```python
from build123d import *

# Parameters (mm, degrees)
SKETCH1_W           = 31
SKETCH1_H           = 16.5
BOSS_EXTRUDE1_DEPTH = 13
SKETCH2_W           = 21
SKETCH2_H           = 1.75
CUT_EXTRUDE1_DEPTH  = 1.6


with BuildPart() as part:
    # Sketch1 → Boss-Extrude1 (new body)
    with BuildSketch(Plane(origin=(0, 0, 0), x_dir=(1, 0, 0), z_dir=(0, 1, 0))):
        Rectangle(SKETCH1_W, SKETCH1_H)
        Polygon((10.5, 5), (-10.5, 5), (-10.5, 6.75), (-14, 6.75), (-14, -6.75), (-10.5, -6.75), (-10.5, -5), (10.5, -5), (10.5, -6.75), (14, -6.75), (14, 6.75), (10.5, 6.75), align=None, mode=Mode.SUBTRACT)
    extrude(amount=BOSS_EXTRUDE1_DEPTH)

    # Sketch2 → Cut-Extrude1 (cut)
    with BuildSketch(Plane.XZ):
        with Locations((0, 5.875)):
            Rectangle(SKETCH2_W, SKETCH2_H)
        with Locations((0, -5.875)):
            Rectangle(SKETCH2_W, SKETCH2_H)
    extrude(amount=-CUT_EXTRUDE1_DEPTH, mode=Mode.SUBTRACT)


solid = part.part
```
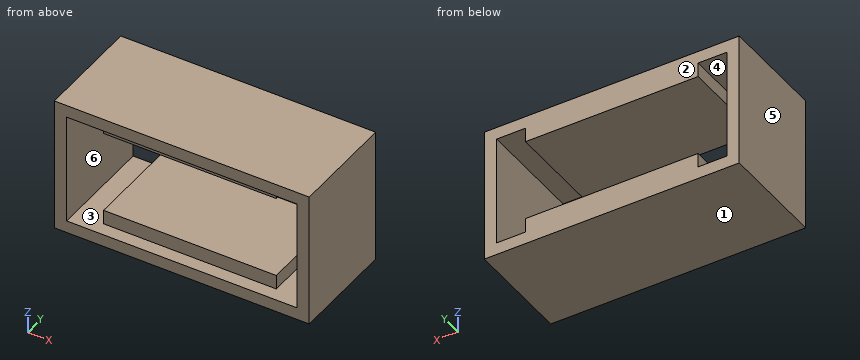
Geometry check sheet. Reference: the model listing, model coordinates, mm. Face numbers are marked on the shaded views. A direction names the side the tool comes from. Round coordinates to 2 decimals unless told otherwise and drop trailing zeros. Loops run counter-clockwise (first coordinate to the right, second up) from the corner with the lowest first, then second, coordinate; pieces in that order, holes last. Notation, with made-up numbers: (12, 37) - (23, 37) arc R25 cw to (23, 58) - close; hole circle Ø10 at (37.25, -11.5). An arc over 180 degrees is marked (long way). Write item = value, one per line. Start each with the question number.
1. Thickness scan on line 1 (X direction, y = 8.75, z = -5.75); line 2 (Z direction, x = -0.5, y = 1.5); line 3 (Z direction, x = 4.5, y = 7). Record the ranges inside material, lowest first.
2. Section check D-D on x = -11. Enter the section's corners in (y, z), then the cut area to 3 significant figures.
3. Section check C-C on y = 9. Enter the section's corners in (x, z), then the cut area to 3 significant figures.
4. Mould release check, pull along Z, two halves, no side actions. Record for the marked faces 1, 2 and 3: released by +Z, released by -Z, zero draft, split by the parting line, or undercut.
5. Set-up check for the marked faces 4, 5 and 6: record each of +Z, -Z, +X, -X, +Y, -Y from which the full face is reachable in a straight line by a thin tool's end or side.
6. Section check A-A on x = 0. Enter the section's corners in (y, z), then the cut area to 3 significant figures.
7. Section check B-B on z = 4.5. Enter the section's corners in (x, y).
8. Depth check by flat-ended pin: pin 1 (1.4 mm diameter, centred on x = 4.5, z = -6, fed in from -Y). Enter the tip coordinate at first touch or a pass-through.
Working result:
q1.line_1 = -15.5 to -14, -10.5 to 10.5, 14 to 15.5
q1.line_2 = -8.25 to -6.75, 6.75 to 8.25
q1.line_3 = -8.25 to -5, 5 to 8.25
q2.outline = (0, -8.25) - (13, -8.25) - (13, -6.75) - (0, -6.75) - close; (0, 6.75) - (13, 6.75) - (13, 8.25) - (0, 8.25) - close
q2.area = 39.0 mm^2
q3.outline = (-15.5, -8.25) - (15.5, -8.25) - (15.5, 8.25) - (-15.5, 8.25) - close; hole (-14, -6.75) - (-10.5, -6.75) - (-10.5, -5) - (10.5, -5) - (10.5, -6.75) - (14, -6.75) - (14, 6.75) - (10.5, 6.75) - (10.5, 5) - (-10.5, 5) - (-10.5, 6.75) - (-14, 6.75) - close
q3.area = 207 mm^2
q4.face_1 = released by -Z
q4.face_2 = zero draft
q4.face_3 = undercut
q5.face_4 = -Y
q5.face_5 = +Z, -Z, -X, +Y, -Y
q5.face_6 = +Y, -Y
q6.outline = (0, -8.25) - (13, -8.25) - (13, -5) - (1.6, -5) - (1.6, -6.75) - (0, -6.75) - close; (0, 6.75) - (1.6, 6.75) - (1.6, 5) - (13, 5) - (13, 8.25) - (0, 8.25) - close
q6.area = 78.9 mm^2
q7.outline = (-15.5, 0) - (-14, 0) - (-14, 13) - (-15.5, 13) - close; (14, 0) - (15.5, 0) - (15.5, 13) - (14, 13) - close
q8.pin_1 = 1.6
